```python
from build123d import *

# Parameters (mm, degrees)
ESBO_O1_W                = 40
ESBO_O1_H                = 40
RESSALTO_EXTRUS_O1_DEPTH = 400
ESBO_O2_W                = 37
ESBO_O2_H                = 37
CORTE_EXTRUS_O1_DEPTH    = 401


with BuildPart() as part:
    # Esboço1 → Ressalto-extrusão1 (new body)
    with BuildSketch(Plane(origin=(0, 0, 0), x_dir=(0, 0, -1), z_dir=(1, 0, 0))):
        Rectangle(ESBO_O1_W, ESBO_O1_H)
    extrude(amount=RESSALTO_EXTRUS_O1_DEPTH)

    # Esboço2 → Corte-extrusão1 (cut, through all)
    with BuildSketch(Plane.ZY):
        Rectangle(ESBO_O2_W, ESBO_O2_H)
    extrude(amount=-CORTE_EXTRUS_O1_DEPTH, mode=Mode.SUBTRACT)


solid = part.part
```
For this review, take the finished solid that the model builds, in its own axes (mm). A direction names the side the tool comes from. Coordinates: 2 decimals unless noted, no trailing zeros. Loops run counter-clockwise (first coordinate to the right, second up) from the corner with the lowest first, then second, coordinate; pieces in that order, holes last. Notation, with made-up numbers: (16, 71.25) -> (62, 71.25) arc R30 ccw to (62, 97.25) -> close; hole circle Ø8 at (-10.5, 80.25). An arc over 180 degrees is marked (long way). Return JSON: item names as keys, results as strings. Group by question number.
(1) Tool access review of faces 5 (the flat face through (197, 0, 18.5)), 6 (the flat face through (197, -20, 0)): name each direction out of +Z, -Z, +X, -X, +Y, -Y from which nothing blocks a thin tool from reaching the whole face with its end or side.
(2) Consider section C-C, the plane x = 331. Give the boundary of the cut face in (y, z).
(3) Mouldability with a two-part tool opening along Z and no side actions: class faces 1 (the flat face through (197, 0, 20)), 2 (the flat face through (197, 18.5, 0)), 3 (the flat face through (400, -19, 2)), 4 (the flat face through (197, 0, -20)) as pulls with the +Z half, pulls with the -Z half, needs draft (parallel to the pull), parting line crosses it, or undercut.
(4) To check wall thickness, follow L1, parallel to Z at x = 178.5, y = -7. State the ranges of the line that lie inside material, in increasing order.
(5) For pin 1 Ø12 at (y, z) = (5.5, -11) entering from -X, flat-tipped, find the tip position at first contact; note if it passes through.
(6) Consider section A-A, the plane y = 10.5. Give the boundary of the cut face in (x, z), plus the area to 3 significant figures.
Results below:
{
 "1": {"face 5": "+X, -X", "face 6": "+Z, -Z, +X, -X, -Y"},
 "2": {"outline": "(-20, -20) -> (20, -20) -> (20, 20) -> (-20, 20) -> close; hole (-18.5, -18.5) -> (18.5, -18.5) -> (18.5, 18.5) -> (-18.5, 18.5) -> close"},
 "3": {"face 1": "pulls with the +Z half", "face 2": "undercut", "face 3": "needs draft", "face 4": "pulls with the -Z half"},
 "4": {"L1": "z = -20 to -18.5, 18.5 to 20"},
 "5": {"pin 1": "passes through"},
 "6": {"outline": "(0, -20) -> (400, -20) -> (400, -18.5) -> (0, -18.5) -> close; (0, 18.5) -> (400, 18.5) -> (400, 20) -> (0, 20) -> close", "area": "1,200 mm2"}
}
